Verification items for this drawing (mm, ordinates from the low corner). A direction names the side the tool comes from. Round coordinates to 2 decimals unless told otherwise and drop trailing zeros. Loops run counter-clockwise (first coordinate to the right, second up) from the corner with the lowest first, then second, coordinate; pieces in that order, holes last. Notation, with made-up numbers: M -39.5,25 L 0.5,25 A11 ccw 0.5,42 Z; hole C 70.25,-3 d1. An arc over 180 degrees is marked long. Write item = value, one per line. Start each with the question number.
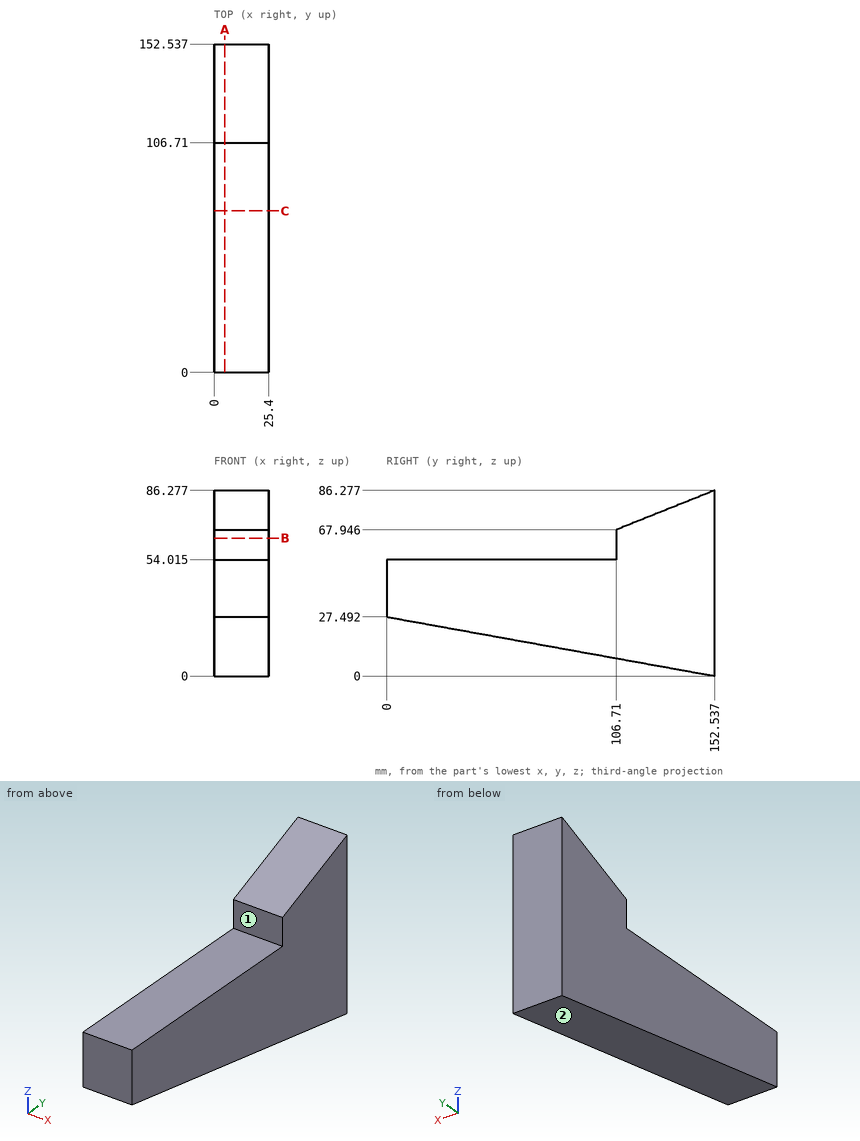
1. Section check B-B, the plane z = 64. Enter the section's corners in (x, y).
2. Tool access check on the marked faces 1 and 2. Record the directions out of +Z, -Z, +X, -X, +Y, -Y that give a thin tool (end or side, any length) a straight path to the whole face; none if there is none.
3. Thickness scan on line 1 (Y direction, x = 7.25, z = 65.5); line 2 (Z direction, x = 3.75, y = 26.5) (1 decimal); line 3 (Z direction, x = 5, y = 44.5) (1 decimal). Record the ranges inside material, lowest first.
4. Section check A-A, the plane x = 5. Enter the section's corners in (y, z) (1 decimal), and give its area (3 significant figures).
5. Gauge pin test, flat ends, axial feed: P1, Ø4, axis at x = 14.5, z = 59, coming from the -Y side; P2, Ø2, axis at x = 20, y = 29.5, coming from the -Z side (1 decimal); P3, Ø8, axis at x = 19.5, y = 135.5, coming from the +Z side. Record the tip position at first contact, or that the pin passes through.
6. Section check C-C, the plane y = 75. Enter the section's corners in (x, z) (1 decimal), and give its area (3 significant figures).
Computed values:
q1.outline = M 0,106.71 L 25.4,106.71 L 25.4,152.54 L 0,152.54 Z
q2.face_1 = +Z, +X, -X, -Y
q2.face_2 = -Z, +X, -X, -Y
q3.line_1 = 106.71 to 152.54
q3.line_2 = 22.7 to 54
q3.line_3 = 19.5 to 54
q4.outline = M 0,27.5 L 152.5,0 L 152.5,86.3 L 106.7,67.9 L 106.7,54 L 0,54 Z
q4.area = 7,200 mm2
q5.P1 = 106.71
q5.P2 = 22
q5.P3 = 81.06
q6.outline = M 0,14 L 25.4,14 L 25.4,54 L 0,54 Z
q6.area = 1,020 mm2
